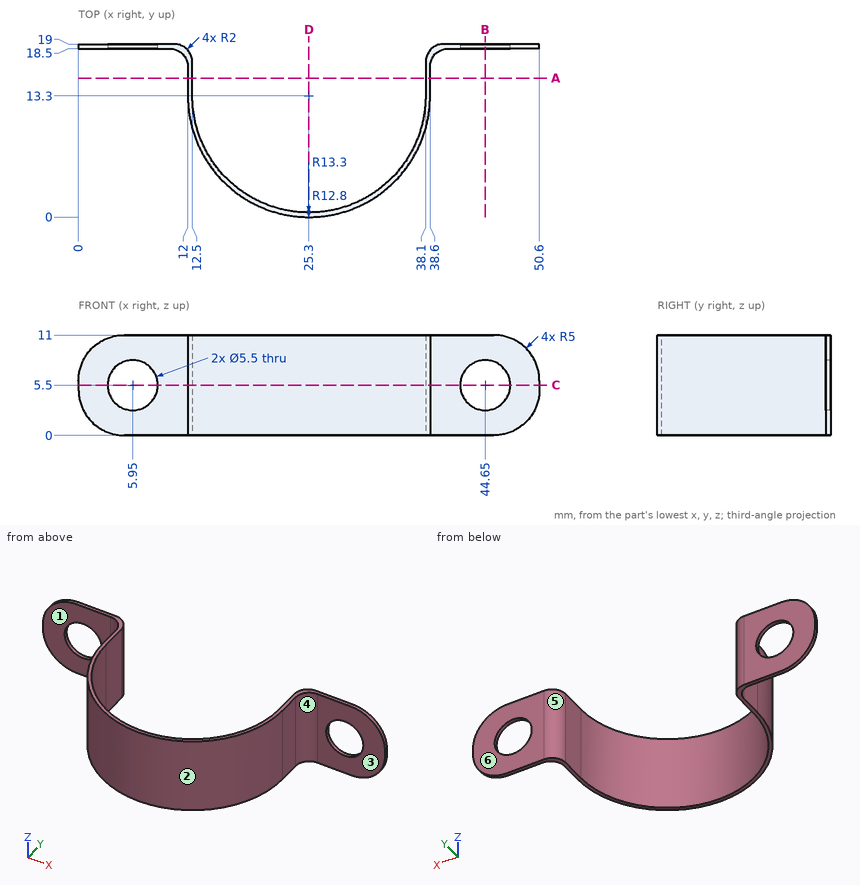
Study the drawing (mm; zero at the part's minimum x, y, z) and answer. A direction names the side the tool comes from. Round coordinates to 2 decimals unless told otherwise and drop trailing zeros. Order: outer loops, then holes, each group sorted by start corner. A loop starts at its lowest first (then second) coordinate and runs counter-clockwise, first axis right, second up. Notation, with made-up numbers: (-6.5, 19.5) -> (16.5, 19.5) arc R12 ccw to (16.5, 41.5) -> close; hole circle Ø11 at (13, 19.25). An arc over 180 degrees is marked (long way). Answer as CSV lines item,"result". Start each with the question number.
(1) The part is cut by section B-B (x = 44.65). Determine the outline of the cut face in (y, z), then the cut area to 3 significant figures.
(2) The part is cut by section C-C (z = 5.5). Determine the outline of the cut face in (x, y).
(3) A tool of negligible diameter and unlimited length cuts with its end or side. For the marked faces 1, 2 and 3, from which of +Z, -Z, +X, -X, +Y, -Y can it reach the whole face along a straight path? Write none if from no direction.
(4) The part is cut by section D-D (x = 25.3). Determine the outline of the cut face in (y, z).
(5) For a pull along X with two mould halves and no side action, classify the marked faces 4, 5 and 6 as +X half, -X half, draft (parallel to the pull), parting line (faces both ways), or undercut.
(6) The part is cut by section A-A (y = 15.25). Determine the outline of the cut face in (x, z), then the cut area to 3 significant figures.
(7) Find the intervals of material crossed by probe 1 along X at (y, z) = (13.75, 5.75); probe 2 along Y at (x, z) = (2, 7.5); probe 3 along Z at (x, y) = (5.95, 18.75), in increasing order. Write a range as from..to.
(8) Flat-ended cylindrical pins translate along their axes: pin 1 Ø1.1 at (y, z) = (15.5, 5.5) entering from +X; pin 2 Ø5 at (x, z) = (4, 3) entering from -Y; pin 3 Ø5 at (x, z) = (44.65, 5.5) entering from +Y; pin 4 Ø1.9 at (y, z) = (15.5, 5.5) entering from -X. Find the tip coordinate at first contact, or state that the pin passes through.
Evaluation:
1,outline,"(18.5, 0) -> (19, 0) -> (19, 2.75) -> (18.5, 2.75) -> close; (18.5, 8.25) -> (19, 8.25) -> (19, 11) -> (18.5, 11) -> close"
1,area,"2.75 mm²"
2,outline,"(0, 18.5) -> (3.2, 18.5) -> (3.2, 19) -> (0, 19) -> close; (8.7, 18.5) -> (10, 18.5) arc R2 cw to (12, 16.5) -> (12, 13.3) arc R13.3 ccw to (38.6, 13.3) -> (38.6, 16.5) arc R2 cw to (40.6, 18.5) -> (41.9, 18.5) -> (41.9, 19) -> (40.1, 19) arc R2 ccw to (38.1, 17) -> (38.1, 13.3) arc R12.8 cw to (12.5, 13.3) -> (12.5, 17) arc R2 ccw to (10.5, 19) -> (8.7, 19) -> close; (47.4, 18.5) -> (50.6, 18.5) -> (50.6, 19) -> (47.4, 19) -> close"
3,face 1,"+Z, -Z, -X, -Y"
3,face 2,"+Z, -Z, -Y"
3,face 3,"+Z, -Z, +X, -Y"
4,outline,"(0, 0) -> (0.5, 0) -> (0.5, 11) -> (0, 11) -> close"
5,face 4,"+X half"
5,face 5,"undercut"
5,face 6,"draft"
6,outline,"(12, 0) -> (12.5, 0) -> (12.5, 11) -> (12, 11) -> close; (38.1, 0) -> (38.6, 0) -> (38.6, 11) -> (38.1, 11) -> close"
6,area,"11.0 mm²"
7,probe 1,"12..12.5, 38.1..38.6"
7,probe 2,"18.5..19"
7,probe 3,"0..2.75, 8.25..11"
8,pin 1,"x = 38.6"
8,pin 2,"y = 18.5"
8,pin 3,"through"
8,pin 4,"x = 12"
